Model file for the job. Use its own axes, mm. A direction names the side the tool comes from. Give positions to 0.01 mm unless a question says otherwise; leave off trailing zeros. Loops run counter-clockwise (first coordinate to the right, second up) from the corner with the lowest first, then second, coordinate; pieces in that order, holes last. Notation, with made-up numbers: M -27,-22 L 20,-22 A23 ccw 20,5 Z; hole C 2.25,7 d10. An arc over 180 degrees is marked long. Answer in a Markdown table with one row per item.
```python
from build123d import *

# Parameters (mm, degrees)
BOSS_EXTRUDE1_DEPTH = 2
SKETCH2_R           = 1.4000000000000001
SKETCH2_R_2         = 1.399999999999999
BOSS_EXTRUDE2_DEPTH = 2
FILLET1_R           = 0.5
BOSS_EXTRUDE3_DEPTH = 5
FILLET2_R           = 2


with BuildPart() as part:
    # Sketch1 → Boss-Extrude1 (new body)
    with BuildSketch(Plane(origin=(0, 0, 0), x_dir=(1, 0, 0), z_dir=(0, 1, 0))):
        Polygon((0, 0), (20, 0), (20, -8), (11.000000000000002, -8), (12, -10), (8.000000000000002, -10), (9.000000000000002, -8), (9.8e-16, -8), align=None)
    extrude(amount=BOSS_EXTRUDE1_DEPTH)

    # Sketch2 → Boss-Extrude2 (add)
    with BuildSketch(Plane(origin=(0, 2, 0), x_dir=(1, 0, 0), z_dir=(0, 1, 0))):
        with Locations(Location((2.3000000000000007, -5.5, 0), (0, 0, 270))):
            Circle(SKETCH2_R)
        with Locations(Location((17.7, -5.499999999999998, 0), (0, 0, 90))):
            Circle(SKETCH2_R_2)
    extrude(amount=BOSS_EXTRUDE2_DEPTH)

    # Fillet1
    fillet1_edges = [part.edges().sort_by_distance(p)[0] for p in [
        (2.3000000000000016, 4, 4.1),
        (17.7, 4, 6.899999999999997),
    ]]
    fillet(fillet1_edges, radius=FILLET1_R)

    # Sketch3 → Boss-Extrude3 (add)
    with BuildSketch(Plane.XZ):
        Polygon((8.000000000000002, 10), (12, 10), (11.000000000000002, 8), (9.000000000000002, 8), align=None)
    extrude(amount=BOSS_EXTRUDE3_DEPTH)

    # Fillet2
    fillet2_edges = [part.edges().sort_by_distance(p)[0] for p in [
        (10.000000000000002, 0, 8),
    ]]
    fillet(fillet2_edges, radius=FILLET2_R)


solid = part.part
```
(1) Saw through at C-C, the plane z = 5.5. Give the cut face in (x, y), and give its area (3 significant figures).
Established:
| item | result |
|---|---|
| outline | M 0,0 L 20,0 L 20,2 L 19.1,2 L 19.1,3.5 A0.5 ccw 18.6,4 L 16.8,4 A0.5 ccw 16.3,3.5 L 16.3,2 L 3.7,2 L 3.7,3.5 A0.5 ccw 3.2,4 L 1.4,4 A0.5 ccw 0.9,3.5 L 0.9,2 L 0,2 Z |
| area | 51.0 mm2 |
(2) Saw through at D-D, the plane y = 1. Give the cut face in (x, z).
Established:
| item | result |
|---|---|
| outline | M 0,0 L 20,0 L 20,8 L 11,8 L 12,10 L 8,10 L 9,8 L 0,8 Z |
(3) Saw through at A-A, the plane x = 17.7. Give the cut face in (y, z), and give its area (3 significant figures).
Established:
| item | result |
|---|---|
| outline | M 0,0 L 2,0 L 2,4.1 L 3.5,4.1 A0.5 ccw 4,4.6 L 4,6.4 A0.5 ccw 3.5,6.9 L 2,6.9 L 2,8 L 0,8 Z |
| area | 21.5 mm2 |
(4) Mould opens along X. For faces 1 (the flat face through (20, 1, 4)), 2 (the cylindrical face through (3.48, 2.74, 6.25)), 3 (the flat face through (18, 4, 6)) say: pulls with the +X half, pulls with the -X half, needs draft (parallel to the pull), parting line crosses it, or undercut.
Established:
| item | result |
|---|---|
| face 1 | pulls with the +X half |
| face 2 | undercut |
| face 3 | needs draft |
(5) Flat gauge pins, fed straight in: P1, Ø1, axis at x = 6.5, z = 3.5, coming from the -Y side; P2, Ø1.6, axis at x = 9.5, y = -4, coming from the -Z side; P3, Ø2, axis at x = 6.5, y = 1, coming from the +Z side. Where does each tip first touch, or does it go through?
Established:
| item | result |
|---|---|
| P1 | stops at y = 0 |
| P2 | stops at z = 8 |
| P3 | stops at z = 8 |
(6) Which spindle directions (+Z, -Z, +X, -X, +Y, -Y) get a long thin tool onto all of the face, cutting with end or side? Do faces 4 (the flat face through (10, -5, 9)), 5 (the flat face through (10, -3, 8)), 6 (the cylindrical face through (19.067, 2.74, 5.803)). Say none if no direction does.
Established:
| item | result |
|---|---|
| face 4 | +Z, -Z, +X, -X, -Y |
| face 5 | -Z, +X, -X, -Y |
| face 6 | +Y |
(7) Wall check: L1, parallel to Y at x = 14.25, z = 7.5; L2, parallel to Z at x = 4, y = 0.25; L3, parallel to Y at x = 2.25, z = 5. Give the ranges that are in metal, low to high.
Established:
| item | result |
|---|---|
| L1 | y = 0 to 2 |
| L2 | z = 0 to 8 |
| L3 | y = 0 to 4 |
(8) Saw through at B-B, the plane y = 2.25. Give the cut face in (x, z), and give its area (3 significant figures).
Established:
| item | result |
|---|---|
| outline | C 2.3,5.5 d2.8; C 17.7,5.5 d2.8 |
| area | 12.3 mm2 |
